For this review, use the dimensioned drawing (mm, ordinates from the lowest corner) and the shaded views. Give positions to 0.01 mm unless a question says otherwise; leave off trailing zeros. Loops run counter-clockwise (first coordinate to the right, second up) from the corner with the lowest first, then second, coordinate; pieces in that order, holes last. Notation, with made-up numbers: (-39.75, 79) - (-12.75, 79) arc R17 cw to (-12.75, 94) - close; hole circle Ø10 at (-2.5, 12.25). An arc over 180 degrees is marked (long way). Write each question's results on one line, items separated by ' | '.
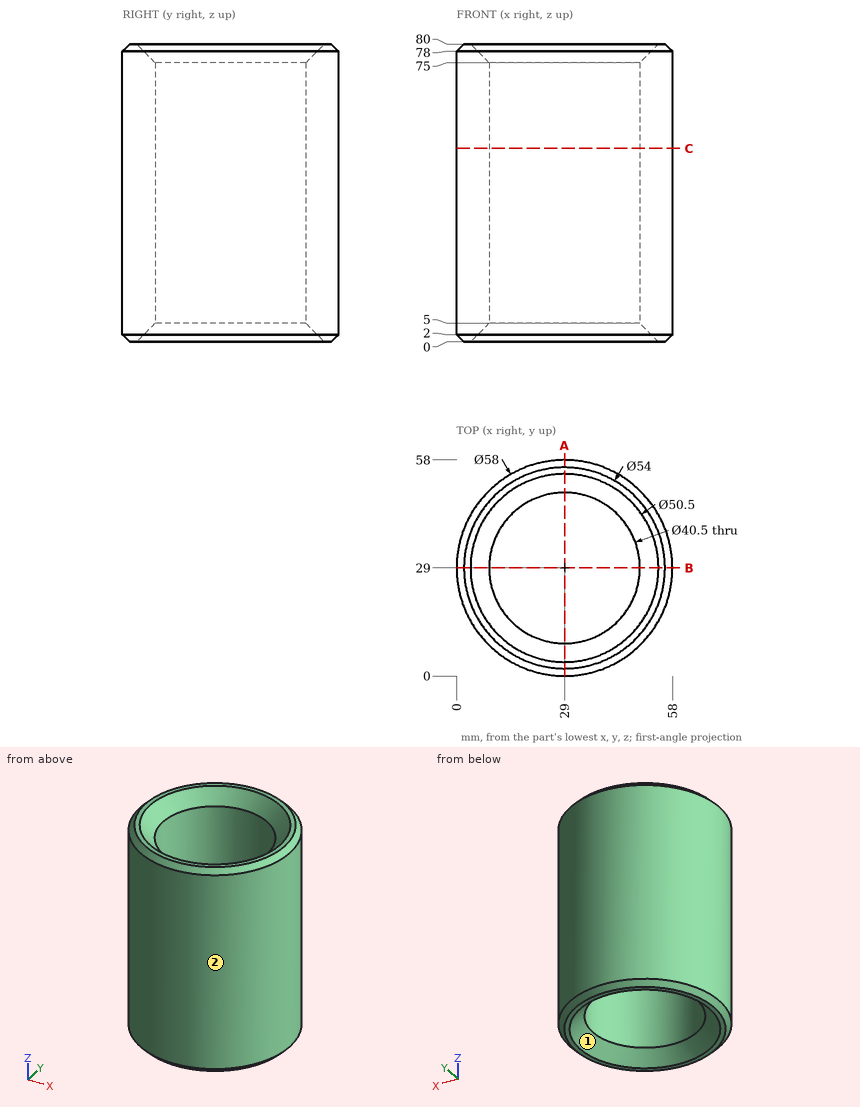
Item 1: Clearance check with flat-ended pins moving along their axes: P1, Ø4, axis at y = 14.5, z = 63, coming from the +X side; P2, Ø4, axis at y = 35, z = 21.5, coming from the +X side; P3, Ø2, axis at x = 44.5, z = 19.5, coming from the -Y side. State where each tip first meets the part, or that it passes through.
Output values:
P1: stops at x = 55.17 | P2: stops at x = 57.72 | P3: stops at y = 3.89
Item 2: We need section A-A on x = 29. Give the boundary of the cut face in (y, z).
Output values:
outline: (0, 2) - (2, 0) - (3.75, 0) - (8.75, 5) - (8.75, 75) - (3.75, 80) - (2, 80) - (0, 78) - close; (49.25, 5) - (54.25, 0) - (56, 0) - (58, 2) - (58, 78) - (56, 80) - (54.25, 80) - (49.25, 75) - close
Item 3: Wall thickness on probe 1 along Y at (x, z) = (29, 51); probe 2 along X at (y, z) = (36, 53); probe 3 along X at (y, z) = (42, 7): over which ranges is each line inside the solid? List them lowest first.
Output values:
probe 1: y = 0 to 8.75, 49.25 to 58 | probe 2: x = 0.86 to 10, 48 to 57.14 | probe 3: x = 3.08 to 13.47, 44.53 to 54.92
Item 4: Draft analysis for pull direction Y (two halves, no side actions). For the marked faces 1 and 2, state which applies: +Y half, -Y half, draft (parallel to the pull), parting line (faces both ways), or undercut.
Output values:
face 1: undercut | face 2: parting line
Item 5: We need section C-C on z = 52. Give the boundary of the cut face in (x, y).
Output values:
outline: circle Ø58 at (29, 29); hole circle Ø40.5 at (29, 29)
